Can you work these out from the model? Positions are in its coordinate system, mm. A direction names the side the tool comes from. Round coordinates to 2 decimals unless told otherwise and drop trailing zeros. Write each loop counter-clockwise with the first axis right and the second up, starting at its lowest first coordinate (ties: lowest second). Pieces come first, ordered by that corner, then holes.
Q1. If we section it at C-C (x = 2.5): Please give me the cut outline in (y, z).
Q2. Please list where these lines run through material, in increasing order: line 1 along X through (y, z) = (-3, 2.75); line 2 along Y through (x, z) = (0, 21.85); line 3 along Y through (x, z) = (3, 15).
Q3. If we section it at B-B (z = 19.25): Please give me the cut outline in (x, y), plus the area to 3 significant figures.
Q4. If we section it at A-A (y = -10.25): Please give me the cut outline in (x, z).
Q5. I'm going to push flat-ended pins straight in: pin 1 Ø5 at (y, z) = (-6, 18.5) entering from +X; pin 2 Ø0.8 at (x, y) = (-27.5, -6) entering from +Z; pin 3 Ø6 at (x, z) = (-7.5, 16.5) entering from +Y; pin 4 Ø0.8 at (x, y) = (0, -3) entering from +Z. Where does each tip first touch, or does it pass through?
Q6. For faces 1 (the flat face through (-28, -6, 4)), 2 (the cylindrical face through (-0.065, -2.504, 22.014)), 3 (the flat face through (22.5, -6, 2)), which set-ups out of +Z, -Z, +X, -X, +Y, -Y let a thin tool reach every point of the face, with its end or its side?
Q7. We'd pull the mould along X, two halves only. Please class faces 4 (the flat face through (28.5, -6, 2)), 5 (the flat face through (-22.5, -6, 2)), 6 (the flat face through (0, 0, 6)): +X half, -X half, draft (parallel to the pull), parting line (faces both ways), or undercut.
Q8. If we section it at D-D (y = -7): Give the number of separate pieces and of enclosed holes in the cut face, plus the area to 3 significant figures.
from build123d import *

# Parameters (mm, degrees)
SALIENTE_EXTRUIR1_DEPTH = 4
REDONDEO1_R             = 5
CROQUIS2_W              = 3
CROQUIS2_H              = 6
SALIENTE_EXTRUIR2_DEPTH = 19
REDONDEO2_START         = -11.5644
REDONDEO2_DEPTH         = 11.5644
REDONDEO2_START_2       = -6
REDONDEO2_2_DEPTH       = 6
REDONDEO2_START_3       = -11.999981249
REDONDEO2_3_DEPTH       = 5.957327692
REDONDEO2_START_4       = 4
REDONDEO2_4_DEPTH       = 20
CROQUIS3_R              = 0.5
CORTAR_EXTRUIR1_DEPTH   = 2
REDONDEO3_R             = 1


with BuildPart() as part:
    # Croquis1 → Saliente-Extruir1 (new body)
    # profile 1 of 4: a face of its own
    with BuildSketch(Plane.XY):
        with BuildLine():
            Line((-21.5, -3.5), (-21.5, -8.5))
            ThreePointArc((-21.5, -8.5), (-25, -12), (-28.5, -8.5))
            Line((-28.5, -8.5), (-28.5, -3.5))
            ThreePointArc((-28.5, -3.5), (-25, 0), (-21.5, -3.5))
        make_face()
        with BuildLine():
            ThreePointArc((-27.5, -8.5), (-25, -11), (-22.5, -8.5))
            Line((-22.5, -8.5), (-22.5, -3.5))
            ThreePointArc((-22.5, -3.5), (-25, -1), (-27.5, -3.5))
            Line((-27.5, -3.5), (-27.5, -8.5))
        make_face(mode=Mode.SUBTRACT)
    # profile 2 of 4: a face of its own
    with BuildSketch(Plane.XY):
        with BuildLine():
            Line((0, 0), (-25, 0))
            ThreePointArc((-25, 0), (-22.525126266, -1.025126266), (-21.5, -3.5))
            Line((-21.5, -3.5), (-21.5, -6))
            Line((-21.5, -6), (0, -6))
            Line((0, -6), (0, 0))
        make_face()
    # profile 3 of 4: a face of its own
    with BuildSketch(Plane.XY):
        with BuildLine():
            Line((25, 0), (0, 0))
            Line((0, 0), (0, -6))
            Line((0, -6), (21.5, -6))
            Line((21.5, -6), (21.5, -3.5))
            ThreePointArc((21.5, -3.5), (22.525126266, -1.025126266), (25, 0))
        make_face()
    # profile 4 of 4: a face of its own
    with BuildSketch(Plane.XY):
        with BuildLine():
            ThreePointArc((28.5, -8.5), (25, -12), (21.5, -8.5))
            Line((21.5, -8.5), (21.5, -3.5))
            ThreePointArc((21.5, -3.5), (25, 0), (28.5, -3.5))
            Line((28.5, -3.5), (28.5, -8.5))
        make_face()
        with BuildLine():
            Line((22.5, -3.5), (22.5, -8.5))
            ThreePointArc((22.5, -8.5), (25, -11), (27.5, -8.5))
            Line((27.5, -8.5), (27.5, -3.5))
            ThreePointArc((27.5, -3.5), (25, -1), (22.5, -3.5))
        make_face(mode=Mode.SUBTRACT)
    extrude(amount=SALIENTE_EXTRUIR1_DEPTH)

    # Redondeo1
    redondeo1_edges = [part.edges().sort_by_distance(p)[0] for p in [
        (21.5, -6, 2),
        (-21.5, -6, 2),
    ]]
    fillet(redondeo1_edges, radius=REDONDEO1_R)

    # Croquis2 → Saliente-Extruir2 (add)
    with BuildSketch(Plane.XY.offset(4)):
        with Locations((0, -3)):
            Rectangle(CROQUIS2_W, CROQUIS2_H)
    extrude(amount=SALIENTE_EXTRUIR2_DEPTH)

    # Redondeo2: read off the stored shape, not the designer's step
    # Redondeo2 outline → Redondeo2 (add)
    with BuildSketch(Plane(origin=(0, 0, 0), x_dir=(1, 0, 0), z_dir=(0, 1, 0)).offset(REDONDEO2_START)):
        with BuildLine():
            ThreePointArc((1.5, -23), (9.10150319, -10.367130938), (22.5, -4.214691199))
            Line((22.5, -4.214691199), (22.5, -4))
            Line((22.5, -4), (1.5, -4))
            Line((1.5, -4), (1.5, -23))
        make_face()
        with BuildLine():
            Line((-22.5, -4), (-22.5, -4.214691199))
            ThreePointArc((-22.5, -4.214691199), (-9.10150319, -10.367130938), (-1.5, -23))
            Line((-1.5, -23), (-1.5, -4))
            Line((-1.5, -4), (-22.5, -4))
        make_face()
    extrude(amount=REDONDEO2_DEPTH)

    # Redondeo2 2 outline → Redondeo2 2 (add)
    with BuildSketch(Plane(origin=(0, 0, 0), x_dir=(1, 0, 0), z_dir=(0, 1, 0)).offset(REDONDEO2_START_2)):
        with BuildLine():
            ThreePointArc((22.5, -4.214691199), (24.131140284, -4.053730539), (25.769322199, -4))
            Line((25.769322199, -4), (22.5, -4))
            Line((22.5, -4), (22.5, -4.214691199))
        make_face()
        with BuildLine():
            Line((-22.5, -4), (-25.769322199, -4))
            ThreePointArc((-25.769322199, -4), (-24.131140284, -4.053730539), (-22.5, -4.214691199))
            Line((-22.5, -4.214691199), (-22.5, -4))
        make_face()
    extrude(amount=REDONDEO2_2_DEPTH)

    # Redondeo2 3 outline → Redondeo2 3 (add)
    with BuildSketch(Plane(origin=(0, 0, 0), x_dir=(1, 0, 0), z_dir=(0, 1, 0)).offset(REDONDEO2_START_3)):
        with BuildLine():
            ThreePointArc((22.5, -4.214691199), (24.131140284, -4.053730539), (25.769322199, -4))
            Line((25.769322199, -4), (22.5, -4))
            Line((22.5, -4), (22.5, -4.214691199))
        make_face()
        with BuildLine():
            Line((-22.5, -4), (-25.769322199, -4))
            ThreePointArc((-25.769322199, -4), (-24.131140284, -4.053730539), (-22.5, -4.214691199))
            Line((-22.5, -4.214691199), (-22.5, -4))
        make_face()
    extrude(amount=REDONDEO2_3_DEPTH)

    # Redondeo2 4 outline → Redondeo2 4 (cut)
    with BuildSketch(Plane.XY.offset(REDONDEO2_START_4)):
        with BuildLine():
            Line((-24.988543271, -11.999981249), (-22.5, -11.999981249))
            Line((-22.5, -11.999981249), (-22.5, -11.5644))
            Line((-22.5, -11.5644), (-1.5, -11.5644))
            Line((-1.5, -11.5644), (-1.5, -6))
            Line((-1.5, -6), (-16.875961595, -6))
            ThreePointArc((-16.875961595, -6), (-19.846404224, -6.978001667), (-21.654807716, -9.529411765))
            ThreePointArc((-21.654807716, -9.529411765), (-22.916085044, -11.311991902), (-24.988543271, -11.999981249))
        make_face()
        with BuildLine():
            Line((-25.769322199, -11.999981249), (-25.011456729, -11.999981249))
            ThreePointArc((-25.011456729, -11.999981249), (-25.392727477, -11.977896653), (-25.769322199, -11.914402342))
            Line((-25.769322199, -11.914402342), (-25.769322199, -11.999981249))
        make_face()
        with BuildLine():
            Line((22.5, -6), (25.769322199, -6))
            Line((25.769322199, -6), (25.769322199, -1.121314785))
            ThreePointArc((25.769322199, -1.121314785), (23.529167837, -1.478452882), (22.5, -3.5))
            Line((22.5, -3.5), (22.5, -6))
        make_face()
        with BuildLine():
            ThreePointArc((22.5, -8.5), (23.529167837, -10.521547118), (25.769322199, -10.878685215))
            Line((25.769322199, -10.878685215), (25.769322199, -6.042653557))
            Line((25.769322199, -6.042653557), (22.5, -6.042653557))
            Line((22.5, -6.042653557), (22.5, -8.5))
        make_face()
        with BuildLine():
            Line((25.011456729, -11.999981249), (25.769322199, -11.999981249))
            Line((25.769322199, -11.999981249), (25.769322199, -11.914402342))
            ThreePointArc((25.769322199, -11.914402342), (25.392727477, -11.977896653), (25.011456729, -11.999981249))
        make_face()
        with BuildLine():
            Line((1.5, -11.5644), (22.5, -11.5644))
            Line((22.5, -11.5644), (22.5, -11.999981249))
            Line((22.5, -11.999981249), (24.988543271, -11.999981249))
            ThreePointArc((24.988543271, -11.999981249), (22.916085044, -11.311991902), (21.654807716, -9.529411765))
            ThreePointArc((21.654807716, -9.529411765), (19.846404224, -6.978001667), (16.875961595, -6))
            Line((16.875961595, -6), (1.5, -6))
            Line((1.5, -6), (1.5, -11.5644))
        make_face()
        with BuildLine():
            ThreePointArc((25, 0), (25.387034755, -0.021465237), (25.769322199, -0.085597658))
            Line((25.769322199, -0.085597658), (25.769322199, 0))
            Line((25.769322199, 0), (25, 0))
        make_face()
        with BuildLine():
            ThreePointArc((-25.769322199, -10.878685215), (-23.529167837, -10.521547118), (-22.5, -8.5))
            Line((-22.5, -8.5), (-22.5, -6.042653557))
            Line((-22.5, -6.042653557), (-25.769322199, -6.042653557))
            Line((-25.769322199, -6.042653557), (-25.769322199, -10.878685215))
        make_face()
        with BuildLine():
            ThreePointArc((-25.769322199, -0.085597658), (-25.387034755, -0.021465237), (-25, 0))
            Line((-25, 0), (-25.769322199, 0))
            Line((-25.769322199, 0), (-25.769322199, -0.085597658))
        make_face()
        with BuildLine():
            Line((-25.769322199, -6), (-22.5, -6))
            Line((-22.5, -6), (-22.5, -3.5))
            ThreePointArc((-22.5, -3.5), (-23.529167837, -1.478452882), (-25.769322199, -1.121314785))
            Line((-25.769322199, -1.121314785), (-25.769322199, -6))
        make_face()
    extrude(amount=REDONDEO2_4_DEPTH, mode=Mode.SUBTRACT)

    # Croquis3 → Cortar-Extruir1 (cut)
    with BuildSketch(Plane.XY.offset(23)):
        with Locations((0, -3)):
            Circle(CROQUIS3_R)
    extrude(amount=-CORTAR_EXTRUIR1_DEPTH, mode=Mode.SUBTRACT)

    # Redondeo3
    redondeo3_edges = [part.edges().sort_by_distance(p)[0] for p in [
        (-1.5, -3, 23),
        (1.5, -3, 23),
    ]]
    fillet(redondeo3_edges, radius=REDONDEO3_R)


solid = part.part
A:
1. outline: (-6, 0) - (0, 0) - (0, 19.86) - (-6, 19.86) - close
2. line 1: x = -28.46 to -27.45, -22.55 to 22.55, 27.45 to 28.46
2. line 2: y = -6 to -3.5, -2.5 to 0
2. line 3: y = -6 to 0
3. outline: (-2.75, -6) - (2.75, -6) - (2.75, 0) - (-2.75, 0) - close
3. area: 33.0 mm2
4. outline: (-28.03, 0) - (-26.79, 0) - (-26.79, 4) - (-28.03, 4) - close; (-23.21, 0) - (-21.97, 0) - (-21.97, 4.29) arc R25 cw to (-23.21, 4.13) - close; (21.97, 0) - (23.21, 0) - (23.21, 4.13) arc R25 cw to (21.97, 4.29) - close; (26.79, 0) - (28.03, 0) - (28.03, 4) - (26.79, 4) - close
5. pin 1: stops at x = 4.42
5. pin 2: stops at z = 4
5. pin 3: stops at y = 0
5. pin 4: stops at z = 21
6. face 1: +Z, -X, +Y, -Y
6. face 2: +Z
6. face 3: +Z, -Z
7. face 4: +X half
7. face 5: undercut
7. face 6: draft
8. separate pieces: 4
8. enclosed holes: 0
8. area: 31.3 mm2
